```python
from build123d import *

# Parameters (mm, degrees)
BOSS_EXTRUDE1_DEPTH      = 3.5
BOSS_EXTRUDE1_DEPTH_BACK = 3.5
CUT_EXTRUDE1_DEPTH       = 3.5
CUT_EXTRUDE1_DEPTH_BACK  = 3.5
SKETCH2_R                = 3


with BuildPart() as part:
    # Sketch1 → Boss-Extrude1 (new, two sides: drawn at the far end of the back side and taken through both)
    with BuildSketch(Plane.XY.offset(-BOSS_EXTRUDE1_DEPTH_BACK)):
        Polygon((0, 25), (0, 18), (5.5, 18), (29.023150547, 23), (29, 23), (30, 24), (30, 34), (29.5, 34), (15, 28), (3, 28), align=None)
    extrude(amount=BOSS_EXTRUDE1_DEPTH + BOSS_EXTRUDE1_DEPTH_BACK)

    # Sketch2 → Cut-Extrude1 (cut, two sides: drawn at the far end of the back side and taken through both)
    with BuildSketch(Plane.XY.offset(-CUT_EXTRUDE1_DEPTH_BACK)):
        with Locations((7.5, 23)):
            Circle(SKETCH2_R)
    extrude(amount=CUT_EXTRUDE1_DEPTH + CUT_EXTRUDE1_DEPTH_BACK, mode=Mode.SUBTRACT)

    # Sketch3 → Cut-Revolve1 (revolve, cut)
    with BuildSketch(Plane.XY, mode=Mode.PRIVATE) as cut_revolve1_sk:
        Polygon((4.901923789, 23), (4.901923789, 21.5), (4.631423789, 21.7705), (0.2705, 21.7705), (0, 21.5), (0, 23), align=None)
    revolve(cut_revolve1_sk.sketch.rotate(Axis((0, 23, 0), (1, 0, 0)), 90), axis=Axis((0, 23, 0), (1, 0, 0)), mode=Mode.SUBTRACT)

    # Sketch4 → Cut-Revolve2 (revolve, cut)
    with BuildSketch(Plane.XY, mode=Mode.PRIVATE) as cut_revolve2_sk:
        Polygon((22.955657634, 25.799676948), (25.401026635, 26.319456175), (26.085657632, 23.098520573), (27.951102449, 21.887086545), (23.967294024, 21.040301924), align=None)
    revolve(cut_revolve2_sk.sketch.rotate(Axis((23.967294024, 21.040301924, 0), (-0.20791169081768215, 0.9781476007338221, 0)), 180), axis=Axis((23.967294024, 21.040301924, 0), (-0.20791169081768215, 0.9781476007338221, 0)), mode=Mode.SUBTRACT)


solid = part.part
```
The listing builds one solid part. Answer for the finished solid, in the listing's coordinates (mm). A direction names the side the tool comes from. Round coordinates to 2 decimals unless told otherwise and drop trailing zeros. Loops run counter-clockwise (first coordinate to the right, second up) from the corner with the lowest first, then second, coordinate; pieces in that order, holes last. Notation, with made-up numbers: (40.5, -5.5) - (47.5, -5.5) arc R20 ccw to (47.5, 18.5) - close; hole circle Ø11 at (68, -22). An arc over 180 degrees is marked (long way). Return JSON: item names as keys, results as strings. Group by question number.
1. The part is cut by section D-D on x = 27.75. Determine the outline of the cut face in (y, z).
2. Each of these flat-tipped pins is pushed along its axis until it touches: P1, Ø3.5, axis at x = 6.5, z = -1, coming from the +Y side; P2, Ø3.5, axis at x = 7.5, y = 23, coming from the +Z side; P3, Ø1.5, axis at y = 30.5, z = -1, coming from the -X side; P4, Ø3, axis at x = 19.5, z = 2.5, coming from the +Y side. Where does it stop, or does it pass through?
3. The mould has two halves that part along X. Classify faces 4 (the flat face through (9, 28, 0)), 5 (the flat face through (29.5, 23.5, 0)), 6 (the cylindrical face through (21.99, 23.89, 2.11)): pulls with the +X half, pulls with the -X half, needs draft (parallel to the pull), parting line crosses it, or undercut.
4. Consider probe 1 along X at (y, z) = (24.25, -1); probe 2 along Y at (x, z) = (7.5, 1.5); probe 3 along Y at (x, z) = (3.45, 0). Determine where each line is inside the solid, lowest interval first.
5. Which of the six approach directions +Z, -Z, +X, -X, +Y, -Y give full straight-line access (tool end or side, diameter ignored) to faces 1 (the cylindrical face through (2.42, 21.91, -0.57)), 2 (the flat face through (15, 24, 3.5)), 3 (the flat face through (22.921, 25.792, 0.035))?
6. The part is cut by section A-A on x = 8.5. Determine the outline of the cut face in (y, z), then the cut area to 3 significant figures.
7. The part is cut by section C-C on y = 27.25. Determine the outline of the cut face in (x, z), then the cut area to 3 significant figures.
Resolved:
{
 "1": {"outline": "(22.73, -3.5) - (33.28, -3.5) - (33.28, 3.5) - (22.73, 3.5) - close"},
 "2": {"P1": "stops at y = 28", "P2": "passes through", "P3": "stops at x = 19.23", "P4": "stops at y = 30.48"},
 "3": {"face 4": "needs draft", "face 5": "pulls with the +X half", "face 6": "undercut"},
 "4": {"probe 1": "x = 0 to 4.77, 10.23 to 20.94, 25.63 to 30", "probe 2": "y = 18.43 to 20, 26 to 28", "probe 3": "y = 18 to 21.77, 24.23 to 28"},
 "5": {"face 1": "-X", "face 2": "+Z, +X, -X, +Y, -Y", "face 3": "none"},
 "6": {"outline": "(18.64, -3.5) - (20.17, -3.5) - (20.17, 3.5) - (18.64, 3.5) - close; (25.83, -3.5) - (28, -3.5) - (28, 3.5) - (25.83, 3.5) - close", "area": "25.9 mm²"},
 "7": {"outline": "(2.25, -3.5) - (30, -3.5) - (30, 3.5) - (2.25, 3.5) - close", "area": "194 mm²"}
}
